Input: part model. Units: mm. Frame: model coordinates. A direction names the side the tool comes from. Give positions to 0.01 mm unless a question says otherwise; leave off trailing zeros. Order: outer loops, then holes, each group sorted by start corner. A loop starts at its lowest first (then second) coordinate and runs counter-clockwise, first axis right, second up. Notation, with made-up numbers: (89, 58.25) - (144, 58.25) arc R15 cw to (144, 72.25) - close; hole circle Ø11 at (-31, -6). An arc over 180 degrees is marked (long way). Use a Markdown table: item, result.
from build123d import *

# Parameters (mm, degrees)
SKETCH_1_W          = 75
SKETCH_1_H          = 75
EXTRUDE_1_DEPTH     = 15
CHAMFER_1_SIZE      = 2
SKETCH_2_R          = 12.5
SKETCH_2_R_2        = 3.25
CUT_EXTRUDE_1_DEPTH = 16
SKETCH_3_R          = 20.25
CUT_EXTRUDE_2_DEPTH = 5


with BuildPart() as part:
    # 草图1 → 凸台-拉伸1 (new body)
    with BuildSketch(Plane.XY):
        with Locations((37.5, -37.5)):
            Rectangle(SKETCH_1_W, SKETCH_1_H)
    extrude(amount=EXTRUDE_1_DEPTH)

    # 倒角1
    chamfer_1_edges = [part.edges().sort_by_distance(p)[0] for p in [
        (0, 0, 7.5),
        (75, 0, 7.5),
        (75, -75, 7.5),
        (0, -75, 7.5),
    ]]
    chamfer(chamfer_1_edges, length=CHAMFER_1_SIZE)

    # 草图2 → 切除-拉伸1 (cut, through all)
    with BuildSketch(Plane.XY.offset(15)):
        with Locations((37.5, -37.5)):
            Circle(SKETCH_2_R)
        with Locations((7.5, -7.5)):
            Circle(SKETCH_2_R_2)
        with Locations((67.5, -7.5)):
            Circle(SKETCH_2_R_2)
        with Locations((67.5, -67.5)):
            Circle(SKETCH_2_R_2)
        with Locations((7.5, -67.5)):
            Circle(SKETCH_2_R_2)
    extrude(amount=-CUT_EXTRUDE_1_DEPTH, mode=Mode.SUBTRACT)

    # 草图3 → 切除-拉伸2 (cut)
    with BuildSketch(Plane.XY.offset(15)):
        with Locations((37.5, -37.5)):
            Circle(SKETCH_3_R)
    extrude(amount=-CUT_EXTRUDE_2_DEPTH, mode=Mode.SUBTRACT)


solid = part.part
1. Pin query (flat end, axial travel): pin 1 (20 mm diameter, centred on x = 38.5, y = -40, fed in from +Z); pin 2 (6 mm diameter, centred on x = 7.5, y = -7.5, fed in from -Z). Return the tip coordinate at first contact, or that it passes through.
Response:
| item | result |
|---|---|
| pin 1 | stops at z = 10 |
| pin 2 | passes through |
2. Section query A-A (y = -67.5). Return loops of the section in (x, z).
Response:
| item | result |
|---|---|
| outline | (0, 0) - (4.25, 0) - (4.25, 15) - (0, 15) - close; (10.75, 0) - (64.25, 0) - (64.25, 15) - (10.75, 15) - close; (70.75, 0) - (75, 0) - (75, 15) - (70.75, 15) - close |
3. Section query D-D (z = 6). Return loops of the section in (x, y), then the cut area to 3 significant figures.
Response:
| item | result |
|---|---|
| outline | (0, -73) - (2, -75) - (73, -75) - (75, -73) - (75, -2) - (73, 0) - (2, 0) - (0, -2) - close; hole circle Ø6.5 at (7.5, -67.5); hole circle Ø6.5 at (7.5, -7.5); hole circle Ø25 at (37.5, -37.5); hole circle Ø6.5 at (67.5, -67.5); hole circle Ø6.5 at (67.5, -7.5) |
| area | 4,990 mm^2 |
4. Set-up query: faces 5 (the face through (48.386, -20.425, 12.535)), 6 (the face through (74, -1, 7)). Return all of +Z, -Z, +X, -X, +Y, -Y with unobstructed straight access to the full face (end or side cutting, diameter ignored); none if empty.
Response:
| item | result |
|---|---|
| face 5 | +Z |
| face 6 | +Z, -Z, +X, +Y |
5. Section query B-B (x = 37.5). Return loops of the section in (y, z), then the cut area to 4 significant figures.
Response:
| item | result |
|---|---|
| outline | (-75, 0) - (-50, 0) - (-50, 10) - (-57.75, 10) - (-57.75, 15) - (-75, 15) - close; (-25, 0) - (0, 0) - (0, 15) - (-17.25, 15) - (-17.25, 10) - (-25, 10) - close |
| area | 672.5 mm^2 |
6. Mould query, pull axis X, two halves, no side actions, for faces 1 (the face through (75, -38, 7)), 2 (the face through (37, -75, 7)), 3 (the face through (46, -28, 10)), 4 (the face through (1, -74, 7)). Classes: pulls with the +X half, pulls with the -X half, needs draft (parallel to the pull), parting line crosses it, or undercut.
Response:
| item | result |
|---|---|
| face 1 | pulls with the +X half |
| face 2 | needs draft |
| face 3 | undercut |
| face 4 | pulls with the -X half |
7. Material intervals for line 1 along Y through (x, z) = (67.5, 3); line 2 along Y through (x, z) = (37.5, 13.1); line 3 along Y through (x, z) = (70, 10.75), sorted ascending.
Response:
| item | result |
|---|---|
| line 1 | y = -75 to -70.75, -64.25 to -10.75, -4.25 to 0 |
| line 2 | y = -75 to -57.75, -17.25 to 0 |
| line 3 | y = -75 to -69.58, -65.42 to -9.58, -5.42 to 0 |
8. Section query C-C (y = -37.5). Return loops of the section in (x, z), then the cut area to 4 significant figures.
Response:
| item | result |
|---|---|
| outline | (0, 0) - (25, 0) - (25, 10) - (17.25, 10) - (17.25, 15) - (0, 15) - close; (50, 0) - (75, 0) - (75, 15) - (57.75, 15) - (57.75, 10) - (50, 10) - close |
| area | 672.5 mm^2 |
